from build123d import *

# Parameters (mm, degrees)
F0_W     = 139
F0_H     = 55
F1_DEPTH = 2.5
F2_W     = 2.3327280719
F2_H     = 23
F2_W_2   = 0.1672719281
F2_W_3   = 0.1289593171
F2_H_2   = 22.8627715209
F3_DEPTH = 2.5
F5_DEPTH = 3
F6_W     = 139
F6_H     = 1.9677817641
F7_DEPTH = 14
F9_D     = 6


with BuildPart() as f1:
    # F0 (on Top) → F1 (new body)
    with BuildSketch(Plane.XY):
        with Locations((3.418983344, 2.2497611304)):
            Rectangle(F0_W, F0_H)
        Polygon((-46.7749163508, -16.9449970126), (-59.4031140208, 24.8976889998), (-51.4031140208, 24.8976889998), (-38.7749163508, -16.9449970126), align=None, mode=Mode.SUBTRACT)
        Polygon((-25.7749595437, -16.9785083988), (-38.4031572137, 24.8641776135), (-30.4031572137, 24.8641776135), (-17.7749595437, -16.9785083988), align=None, mode=Mode.SUBTRACT)
        Polygon((-4.7749595437, -17.1519126743), (-17.4031572137, 24.6907733381), (-9.4031572137, 24.6907733381), (3.2250404563, -17.1519126743), align=None, mode=Mode.SUBTRACT)
        Polygon((16.2250404563, -17.1519108117), (3.5968427863, 24.6907752007), (11.5968427863, 24.6907752007), (24.2250404563, -17.1519108117), align=None, mode=Mode.SUBTRACT)
        Polygon((37.2244375112, -17.277115479), (24.5962398412, 24.5655705334), (32.5962398412, 24.5655705334), (45.2244375112, -17.277115479), align=None, mode=Mode.SUBTRACT)
        Polygon((58.2235167211, -17.1223909005), (45.5953190511, 24.7202951119), (53.5953190511, 24.7202951119), (66.2235167211, -17.1223909005), align=None, mode=Mode.SUBTRACT)
    extrude(amount=F1_DEPTH)

    # F2 (on face) → F3 (join)
    with BuildSketch(Plane.XZ.offset(25.2502388696)):
        Polygon((-66.081016656, 13.302537529), (-66.081016656, 0), (73.1178743134, 0), (73.1178743134, 13.4397660082), (72.9889149964, 13.4397660082), (72.9889149964, 36.302537529), (-65.9137447279, 36.302537529), (-65.9137447279, 13.302537529), align=None)
        Polygon((-27.6715531448, 14.3061928175), (-35.129489078, 14.3061928175), (-34.4548327198, 17.8079805818), (-26.9968967865, 17.8079805818), align=None, mode=Mode.SUBTRACT)
        Polygon((-38.5440763607, 8.4408130497), (-55.0066094022, 8.4408130497), (-51.0917667246, 28.6483773044), (-35.2029210626, 28.6483773044), (-35.8316824305, 25.3806539909), (-47.4935994805, 25.3806539909), (-48.4849312723, 20.3000785582), (-37.6996085381, 20.3000785582), (-38.328369906, 17.0323552447), (-49.1136926402, 17.0323552447), (-50.1463299232, 11.7131258622), (-37.8969569966, 11.7131258622), align=None, mode=Mode.SUBTRACT)
        with BuildLine():
            Line((-5.0958073876, 8.4408130497), (-8.8546070979, 8.4408130497))
            Line((-8.8546070979, 8.4408130497), (-6.3900461157, 21.1215988857))
            add(Edge.make_bspline(
                [(-6.3900461157, 21.1215988857), (-6.0137071947, 22.9849354942), (-5.3252823394, 25.7386349157)],
                knots=[0, 0, 0, 1, 1, 1], degree=2))
            Line((-5.3252823394, 25.7386349157), (-6.3166141311, 23.5723913708))
            add(Edge.make_bspline(
                [(-6.3166141311, 23.5723913708), (-7.450220393, 21.0757038953), (-7.9504757879, 20.144035591)],
                knots=[0, 0, 0, 1, 1, 1], degree=2))
            Line((-7.9504757879, 20.144035591), (-13.861750546, 8.4408130497))
            Line((-13.861750546, 8.4408130497), (-16.8724619135, 8.4408130497))
            Line((-16.8724619135, 8.4408130497), (-18.22177463, 20.1853410823))
            add(Edge.make_bspline(
                [(-18.22177463, 20.1853410823), (-18.6669560365, 24.3617852049), (-18.7954620095, 25.7386349157)],
                knots=[0, 0, 0, 1, 1, 1], degree=2))
            add(Edge.make_bspline(
                [(-18.7954620095, 25.7386349157), (-19.1947484256, 22.2368471514), (-19.4104548803, 21.162904377)],
                knots=[0, 0, 0, 1, 1, 1], degree=2))
            Line((-19.4104548803, 21.162904377), (-21.8796053616, 8.4408130497))
            Line((-21.8796053616, 8.4408130497), (-25.6338155729, 8.4408130497))
            Line((-25.6338155729, 8.4408130497), (-21.7052043982, 28.6483773044))
            Line((-21.7052043982, 28.6483773044), (-16.041762588, 28.6483773044))
            Line((-16.041762588, 28.6483773044), (-14.7796503532, 17.3490306782))
            Line((-14.7796503532, 17.3490306782), (-14.4216694284, 13.3882930103))
            add(Edge.make_bspline(
                [(-14.4216694284, 13.3882930103), (-13.9030560373, 14.5356677692), (-13.4578746309, 15.4673360735)],
                knots=[0, 0, 0, 1, 1, 1], degree=2))
            add(Edge.make_bspline(
                [(-13.4578746309, 15.4673360735), (-13.0126932244, 16.3990043778), (-6.8031010289, 28.6483773044)],
                knots=[0, 0, 0, 1, 1, 1], degree=2))
            Line((-6.8031010289, 28.6483773044), (-1.1671962129, 28.6483773044))
            Line((-1.1671962129, 28.6483773044), (-5.0958073876, 8.4408130497))
        make_face(mode=Mode.SUBTRACT)
        Polygon((17.401916886, 8.4408130497), (13.2162937654, 8.4408130497), (12.4268999312, 13.603999465), (4.7257205491, 13.603999465), (1.9307156363, 8.4408130497), (-2.2870339777, 8.4408130497), (8.9985441514, 28.6483773044), (13.9919191024, 28.6483773044), align=None, mode=Mode.SUBTRACT)
        Polygon((27.5309412581, 18.9966608321), (22.6844302763, 28.6483773044), (27.1132968458, 28.6483773044), (30.3259461709, 21.8926347237), (36.0903569599, 28.6483773044), (40.583476516, 28.6483773044), (31.9781658238, 18.9415868436), (37.2377317189, 8.4408130497), (32.8364021435, 8.4408130497), (29.2061084062, 16.0731499462), (22.6844302763, 8.4408130497), (18.1775422231, 8.4408130497), align=None, mode=Mode.SUBTRACT)
        Polygon((47.123512642, 18.9966608321), (42.2770016602, 28.6483773044), (46.7058682298, 28.6483773044), (49.9185175548, 21.8926347237), (55.6829283438, 28.6483773044), (60.1760478999, 28.6483773044), (51.5707372077, 18.9415868436), (56.8303031028, 8.4408130497), (52.4289735274, 8.4408130497), (48.7986797901, 16.0731499462), (42.2770016602, 8.4408130497), (37.770113607, 8.4408130497), align=None, mode=Mode.SUBTRACT)
        with Locations((-67.247380692, 24.802537529)):
            Rectangle(F2_W, F2_H)
        with Locations((-65.997380692, 24.802537529)):
            Rectangle(F2_W_2, F2_H)
        with Locations((73.0533946549, 24.8711517686)):
            Rectangle(F2_W_3, F2_H_2)
        Polygon((73.1178743134, 36.302537529), (73.1178743134, 13.4397660082), (75.4889149964, 13.4397660082), (75.4889149964, 36.4397660082), (72.9889149964, 36.4397660082), (72.9889149964, 36.302537529), align=None)
    extrude(amount=F3_DEPTH)

    # F4 (on face) → F5 (join)
    with BuildSketch(Plane(origin=(0, 0, 13.4397660082), x_dir=(1, 0, 0), z_dir=(0, 0, -1))):
        with BuildLine():
            Line((75.4889149964, 25.2502388696), (75.4889149964, 27.7502388696))
            Line((75.4889149964, 27.7502388696), (73.1178743134, 27.7502388696))
            Line((73.1178743134, 27.7502388696), (73.1178743134, 25.2502388696))
            Line((73.1178743134, 25.2502388696), (73.0357726252, -2.464520624))
            ThreePointArc((73.0357726252, -2.464520624), (74.1664237205, -1.6173558789), (75.4889149964, -1.1202876444))
            Line((75.4889149964, -1.1202876444), (75.4889149964, 25.2502388696))
        make_face()
        with BuildLine():
            ThreePointArc((81.5691593623, -6.0022003956), (79.6995569545, -2.1034043102), (75.4889149964, -1.1202876444))
            Line((75.4889149964, -1.1202876444), (75.4889149964, -10.8841131467))
            ThreePointArc((75.4889149964, -10.8841131467), (79.6995569545, -9.9009964809), (81.5691593623, -6.0022003956))
        make_face()
        with BuildLine():
            Line((75.4889149964, -10.8841131467), (75.4889149964, -1.1202876444))
            ThreePointArc((75.4889149964, -1.1202876444), (74.1664237205, -1.6173558789), (73.0357726252, -2.464520624))
            Line((73.0357726252, -2.464520624), (73.014874911, -9.5188837818))
            ThreePointArc((73.014874911, -9.5188837818), (74.1534447384, -10.3799078842), (75.4889149964, -10.8841131467))
        make_face()
        with BuildLine():
            Line((75.4889149964, -30.0022003956), (75.4889149964, -10.8841131467))
            ThreePointArc((75.4889149964, -10.8841131467), (74.1534447384, -10.3799078842), (73.014874911, -9.5188837818))
            Line((73.014874911, -9.5188837818), (72.9604437947, -27.8929919004))
            Line((72.9604437947, -27.8929919004), (61.0808953643, -27.8929919004))
            Line((61.0808953643, -27.8929919004), (61.0808953643, -30.0022003956))
            Line((61.0808953643, -30.0022003956), (75.4889149964, -30.0022003956))
        make_face()
        with BuildLine():
            Line((73.014874911, -9.5188837818), (73.0357726252, -2.464520624))
            ThreePointArc((73.0357726252, -2.464520624), (71.5691813014, -5.9873885535), (73.014874911, -9.5188837818))
        make_face()
        with BuildLine():
            Line((-68.1669373373, 27.6543483512), (-68.3165375451, 27.5479025488))
            Line((-68.3165375451, 27.5479025488), (-68.3165375451, -0.8886232584))
            ThreePointArc((-68.3165375451, -0.8886232584), (-66.8972077442, -1.452270315), (-65.714216699, -2.4180483823))
            Line((-65.714216699, -2.4180483823), (-65.7958966544, 25.1543483512))
            Line((-65.7958966544, 25.1543483512), (-65.7958966544, 27.6543483512))
            Line((-65.7958966544, 27.6543483512), (-68.1669373373, 27.6543483512))
        make_face()
        with BuildLine():
            ThreePointArc((-65.714216699, -2.4180483823), (-66.8972077442, -1.452270315), (-68.3165375451, -0.8886232584))
            Line((-68.3165375451, -0.8886232584), (-68.3165375451, -10.637216093))
            ThreePointArc((-68.3165375451, -10.637216093), (-66.884449129, -10.0660451489), (-65.6944645318, -9.0857135021))
            Line((-65.6944645318, -9.0857135021), (-65.714216699, -2.4180483823))
        make_face()
        with BuildLine():
            Line((-68.3165375451, -10.637216093), (-68.3165375451, -0.8886232584))
            ThreePointArc((-68.3165375451, -0.8886232584), (-74.4306445579, -5.7629196757), (-68.3165375451, -10.637216093))
        make_face()
        with BuildLine():
            ThreePointArc((-65.6944645318, -9.0857135021), (-66.884449129, -10.0660451489), (-68.3165375451, -10.637216093))
            Line((-68.3165375451, -10.637216093), (-68.3165375451, -29.7629196757))
            Line((-68.3165375451, -29.7629196757), (-53.7589177052, -29.8940964603))
            Line((-53.7589177052, -29.8940964603), (-53.7589177052, -27.9888824189))
            Line((-53.7589177052, -27.9888824189), (-61.1505493085, -27.9888824189))
            Line((-61.1505493085, -27.9888824189), (-65.6384661357, -27.9888824189))
            Line((-65.6384661357, -27.9888824189), (-65.6944645318, -9.0857135021))
        make_face()
        with BuildLine():
            ThreePointArc((-64.4306445579, -5.7629196757), (-64.7625539796, -3.9715709233), (-65.714216699, -2.4180483823))
            Line((-65.714216699, -2.4180483823), (-65.6944645318, -9.0857135021))
            ThreePointArc((-65.6944645318, -9.0857135021), (-64.7572678274, -7.5404319639), (-64.4306445579, -5.7629196757))
        make_face()
    extrude(amount=-F5_DEPTH)

    # F6 (on face) → F7 (join)
    with BuildSketch(Plane.XY.offset(2.5)):
        with Locations((3.5998241897, 28.7658702483)):
            Rectangle(F6_W, F6_H)
    extrude(amount=F7_DEPTH)

    # F9 (through all)
    with Locations(Plane.XY.offset(16.4397660082)):
        with Locations((-69.4306445579, 5.7629196757), (76.5447840095, 5.7629196757)):
            Hole(F9_D / 2)


solid = f1.part
For this review, take the finished solid that the model builds, in its own axes (mm). A direction names the side the tool comes from. Round coordinates to 2 decimals unless told otherwise and drop trailing zeros. Order: outer loops, then holes, each group sorted by start corner. A loop starts at its lowest first (then second) coordinate and runs counter-clockwise, first axis right, second up. Notation, with made-up numbers: M 25,45.5 L 50,45.5 A13 ccw 50,50.5 Z; hole C 11,-9 d7. An arc over 180 degrees is marked long. Write each question's results on one line, items separated by ' | '. Start each with the question number.
1. Add section C-C (y = -21). State the section outline as (x, z) points, then the cut area to 3 significant figures.
2. Clearance check with flat-ended pins moving along their axes: pin 1 Ø2 at (x, y) = (-46.5, -27) entering from -Z; pin 2 Ø5 at (y, z) = (9, 14) entering from +X; pin 3 Ø10 at (x, y) = (-45, 10.5) entering from +Z; pin 4 Ø3 at (x, y) = (7, -26.5) entering from +Z. State where each tip first meets the part, or that it passes through.
3. Add section B-B (x = 69.5). State the section outline as (y, z) points.
4. To check wall thickness, follow L1, parallel to X at y = 27.5, z = 13.5; L2, parallel to Y at x = 31, z = 3.5; L3, parallel to X at y = 22, z = 15. State the ranges of each line that lie inside material, in increasing order. Write a range as [from, to].
5. Add section A-A (x = 6.5). State the section outline as (y, z) points.
6. Draft analysis for pull direction X (two halves, no side actions). For faces 4 (the face through (3, 1, 0)), 5 (the face through (31, 3.35, 1.23)), 6 (the face through (-11, 3.48, 1.23)), state which applies: pulls with the +X half, pulls with the -X half, needs draft (parallel to the pull), parting line crosses it, or undercut.
7. Tool access review of faces 1 (the face through (59.82, 4.09, 1.23)), 2 (the face through (44.734, -26.483, 23.755)), 3 (the face through (15.673, -26.483, 18.686)): name each direction out of +Z, -Z, +X, -X, +Y, -Y from which nothing blocks a thin tool from reaching the whole face with its end or side.
8. Add section D-D (y = -15). State how many separate pieces and enclosed holes the cut face has, then the cut area to 3 significant figures.
Output values:
1) outline: M -68.32,13.44 L -65.78,13.44 L -65.78,16.44 L -68.32,16.44 Z; M -66.08,0 L 72.92,0 L 72.92,2.5 L -66.08,2.5 Z; M 73.11,13.44 L 75.49,13.44 L 75.49,16.44 L 73.11,16.44 Z | area: 362 mm^2
2) pin 1: z = 0 | pin 2: x = 81.54 | pin 3: z = 2.5 | pin 4: z = 36.3
3) outline: M -27.75,0 L 29.75,0 L 29.75,13.44 L 30,13.44 L 30,16.44 L 29.75,16.44 L 29.75,16.5 L 27.78,16.5 L 27.78,2.5 L -25.25,2.5 L -25.25,36.3 L -27.75,36.3 Z
4) L1: [-68.32, -65.64], [72.96, 75.49] | L2: [-27.75, -25.25], [27.78, 29.75] | L3: [-68.32, -65.66], [72.98, 75.49]
5) outline: M -27.75,0 L 15.07,0 L 15.07,2.5 L -25.25,2.5 L -25.25,13.6 L -27.75,13.6 Z; M -27.75,24.17 L -25.25,24.17 L -25.25,36.3 L -27.75,36.3 Z; M 24.69,0 L 29.75,0 L 29.75,16.5 L 27.78,16.5 L 27.78,2.5 L 24.69,2.5 Z
6) face 4: needs draft | face 5: undercut | face 6: undercut
7) face 1: +Z, -Z | face 2: +Y, -Y | face 3: -Y
8) separate pieces: 9 | enclosed holes: 0 | area: 242 mm^2
